The model under review builds one solid part; all positions refer to its coordinate system, in mm. Round coordinates to 2 decimals unless told otherwise and drop trailing zeros. Order: outer loops, then holes, each group sorted by start corner. A loop starts at its lowest first (then second) coordinate and runs counter-clockwise, first axis right, second up. Notation, with made-up numbers: M 11.5,74 L 45.5,74 A26 ccw 45.5,96 Z; hole C 63.5,40 d4. An arc over 180 degrees is marked long. Answer as a JSON object with one key per item and string values. Group by question number.
1. Add section C-C on x = -13.5. State the section outline as (y, z) points.
2. Add section B-B on z = 2.5. State the section outline as (x, y) points.
3. Add section A-A on y = 33. State the section outline as (x, z) points, and give its area (3 significant figures).
4. To check wall thickness, follow probe 1 along Y at (x, z) = (-51.5, 5); probe 2 along X at (y, z) = (14.5, 1.5); probe 3 along X at (y, z) = (-13, 4). State the ranges of each line that lie inside material, in increasing order. Write a range as [from, to].
5. Add section D-D on x = -59.5. State the section outline as (y, z) points.
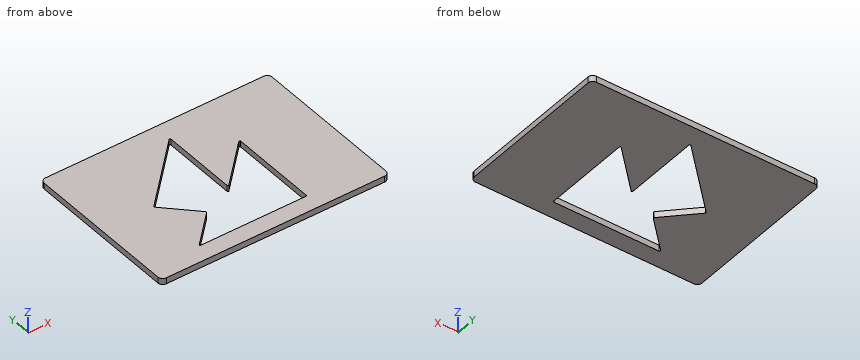
```python
from build123d import *

# Parameters (mm, degrees)
F0_W     = 238.125
F0_H     = 168.275
F1_DEPTH = 6.35
F2_R     = 5.08
F4_DEPTH = 25.4
F6_DEPTH = 6.351


with BuildPart() as f1:
    # F0 (on Top) → F1 (new body)
    with BuildSketch(Plane.XY):
        Rectangle(F0_W, F0_H)
    extrude(amount=F1_DEPTH)

    # F2
    f2_edges = [f1.edges().sort_by_distance(p)[0] for p in [
        (119.0625, -84.1375, 3.175),
        (-119.0625, -84.1375, 3.175),
        (119.0625, 84.1375, 3.175),
        (-119.0625, 84.1375, 3.175),
    ]]
    fillet(f2_edges, radius=F2_R)

    # F3 (on face) → F4 (cut)
    with BuildSketch(Plane.XY.offset(6.35)):
        Polygon((-31.75, -33.3375), (-63.5, -65.0875), (44.958, -65.0875), (44.958, 24.8285), (0, -20.1295), (0, 61.9125), (-63.5, -1.5875), align=None)
    extrude(amount=-F4_DEPTH, mode=Mode.SUBTRACT)

    # F5 (on face) → F6 (cut, through all)
    with BuildSketch(Plane.XY.offset(6.35)):
        with BuildLine():
            ThreePointArc((46.228, 25.993599), (45.741925, 26.721062), (44.883824, 26.550375))
            Line((44.883824, 26.550375), (2.614176, -15.719273))
            ThreePointArc((2.614176, -15.719273), (1.756075, -15.88996), (1.27, -15.162497))
            Line((1.27, -15.162497), (1.27, 63.077599))
            ThreePointArc((1.27, 63.077599), (0.783925, 63.805062), (-0.074176, 63.634375))
            Line((-0.074176, 63.634375), (-64.739275, -1.030724))
            ThreePointArc((-64.739275, -1.030724), (-64.969899, -1.5875), (-64.739275, -2.144276))
            Line((-64.739275, -2.144276), (-34.102827, -32.780724))
            ThreePointArc((-34.102827, -32.780724), (-33.872203, -33.3375), (-34.102827, -33.894276))
            Line((-34.102827, -33.894276), (-65.221875, -65.013324))
            ThreePointArc((-65.221875, -65.013324), (-65.392562, -65.871425), (-64.665099, -66.3575))
            Line((-64.665099, -66.3575), (45.4406, -66.3575))
            ThreePointArc((45.4406, -66.3575), (45.997376, -66.126876), (46.228, -65.5701))
            Line((46.228, -65.5701), (46.228, 25.993599))
        make_face()
    extrude(amount=-F6_DEPTH, mode=Mode.SUBTRACT)


solid = f1.part
```
Recorded:
{
 "1": {"outline": "M -84.14,0 L -66.36,0 L -66.36,6.35 L -84.14,6.35 Z; M 50.21,0 L 84.14,0 L 84.14,6.35 L 50.21,6.35 Z"},
 "2": {"outline": "M -119.06,-79.06 A5.08 ccw -113.98,-84.14 L 113.98,-84.14 A5.08 ccw 119.06,-79.06 L 119.06,79.06 A5.08 ccw 113.98,84.14 L -113.98,84.14 A5.08 ccw -119.06,79.06 Z; hole M -65.22,-65.01 A0.79 ccw -64.67,-66.36 L 45.44,-66.36 A0.79 ccw 46.23,-65.57 L 46.23,25.99 A0.79 ccw 44.88,26.55 L 2.61,-15.72 A0.79 cw 1.27,-15.16 L 1.27,63.08 A0.79 ccw -0.07,63.63 L -64.74,-1.03 A0.79 ccw -64.74,-2.14 L -34.1,-32.78 A0.79 cw -34.1,-33.89 Z"},
 "3": {"outline": "M -119.06,0 L -30.71,0 L -30.71,6.35 L -119.06,6.35 Z; M 1.27,0 L 119.06,0 L 119.06,6.35 L 1.27,6.35 Z", "area": "1,310 mm²"},
 "4": {"probe 1": "y = [-84.14, -66.36], [-51.29, -15.38], [12.21, 84.14]", "probe 2": "x = [-119.06, -49.21], [1.27, 32.83], [46.23, 119.06]", "probe 3": "x = [-119.06, -53.88], [1.27, 5.33], [46.23, 119.06]"},
 "5": {"outline": "M -84.14,0 L -66.36,0 L -66.36,6.35 L -84.14,6.35 Z; M -59.29,0 L -7.38,0 L -7.38,6.35 L -59.29,6.35 Z; M 4.21,0 L 84.14,0 L 84.14,6.35 L 4.21,6.35 Z"}
}
